Can you work these out from the model? Positions are in its coordinate system, mm. A direction names the side the tool comes from. Coordinates: 2 decimals unless noted, no trailing zeros. Order: outer loops, then holes, each group sorted by start corner. A loop starts at its lowest first (then second) coordinate and runs counter-clockwise, first axis right, second up. Notation, with made-up numbers: (-32, 20.5) - (5, 20.5) arc R19 ccw to (5, 53.5) - close; hole circle Ø3 at (-24, 21). An arc over 180 degrees is marked (long way). Use a Markdown table: item, result. Add a question column.
(1) I want a section at D-D (z = -1). List the corners of the cut face in (x, y) for me.
(2) For pin 1 Ø1.5 at (y, z) = (1.5, 2) entering from -X; pin 2 Ø1 at (x, z) = (2, 1.5) entering from +Y; pin 3 Ø1 at (x, z) = (1, -7) entering from -Y, each with a flat end and sliding along its axis, tell me the tip position at first contact or that it passes through.
(3) If I drill on L1, parallel to Z at x = 3, y = -3; L2, parallel to Z at x = -0.25, y = 0.25; L3, parallel to Y at x = -1.5, z = -1, over which ranges is the centre line in solid material (lowest first)? Write a range as [from, to].
(4) I want a section at A-A (z = 0.75). List the corners of the cut face in (x, y) for me.
(5) On a 3-axis mill with a long thin cutter (end or side, diameter ignored), from which of +Z, -Z, +X, -X, +Y, -Y can I reach the whole of each face in a straight line? I mean faces 4 (the flat face through (-1.74, 0.99, 2.46)), 5 (the cylindrical face through (-0.54, -2.44, -4.93)), 6 (the flat face through (0, 0, -10)). Say none if no direction works.
(6) We'd pull the mould along X, two halves only. Please class faces 1 (the flat face through (2, -2, 0)), 2 (the flat face through (0, -2, 2)), 3 (the cylindrical face through (-0.943, -4.247, 2.465)): pulls with the +X half, pulls with the -X half, needs draft (parallel to the pull), parting line crosses it, or undercut.
(7) I want a section at B-B (x = 0). List the corners of the cut face in (y, z) for me.
(8) I want a section at C-C (y = 2.25). List the corners of the cut face in (x, z) for me, and give its area (3 significant figures).
```python
from build123d import *

# Parameters (mm, degrees)
F0_R     = 2.5
F1_DEPTH = 10
F0_R_2   = 4.35
F2_DEPTH = 5


with BuildPart() as f1:
    # F0 (on Top) → F1 (new body)
    with BuildSketch(Plane.XY):
        Circle(F0_R)
        Polygon((2.309401, 0), (1.154701, -2), (-1.154701, -2), (-2.309401, 0), (-1.154701, 2), (1.154701, 2), align=None, mode=Mode.SUBTRACT)
        Polygon((-1.154701, -2), (1.154701, -2), (2.309401, 0), (1.154701, 2), (-1.154701, 2), (-2.309401, 0), align=None)
    extrude(amount=-F1_DEPTH)

    # F0 (on Top) → F2 (join)
    with BuildSketch(Plane.XY):
        Circle(F0_R_2)
        Circle(F0_R, mode=Mode.SUBTRACT)
        Circle(F0_R)
        Polygon((2.309401, 0), (1.154701, -2), (-1.154701, -2), (-2.309401, 0), (-1.154701, 2), (1.154701, 2), align=None, mode=Mode.SUBTRACT)
    extrude(amount=F2_DEPTH)


solid = f1.part
```
Answers follow:
| question | item | result |
|---|---|---|
| 1 | outline | circle Ø5 at (0, 0) |
| 2 | pin 1 | stops at x = -4.28 |
| 2 | pin 2 | stops at y = 4.08 |
| 2 | pin 3 | stops at y = -2.45 |
| 3 | L1 | z = [0, 5] |
| 3 | L2 | z = [-10, 0] |
| 3 | L3 | y = [-2, 2] |
| 4 | outline | circle Ø8.7 at (0, 0); hole (-2.31, 0) - (-1.15, -2) - (1.15, -2) - (2.31, 0) - (1.15, 2) - (-1.15, 2) - close |
| 5 | face 4 | +Z |
| 5 | face 5 | -Z |
| 5 | face 6 | -Z, +X, -X, +Y, -Y |
| 6 | face 1 | needs draft |
| 6 | face 2 | undercut |
| 6 | face 3 | parting line crosses it |
| 7 | outline | (-4.35, 0) - (-2.5, 0) - (-2.5, -10) - (2.5, -10) - (2.5, 0) - (4.35, 0) - (4.35, 5) - (2, 5) - (2, 0) - (-2, 0) - (-2, 5) - (-4.35, 5) - close |
| 8 | outline | (-3.72, 0) - (-1.09, 0) - (-1.09, -10) - (1.09, -10) - (1.09, 0) - (3.72, 0) - (3.72, 5) - (-3.72, 5) - close |
| 8 | area | 59.0 mm² |
